Input: part model. Units: mm. Frame: model coordinates. A direction names the side the tool comes from. Round coordinates to 2 decimals unless told otherwise and drop trailing zeros. Loops run counter-clockwise (first coordinate to the right, second up) from the corner with the lowest first, then second, coordinate; pieces in that order, holes last. Notation, with made-up numbers: (84.5, 48.25) -> (125.5, 48.25) arc R13 ccw to (125.5, 57.25) -> close; hole circle Ø1 at (27.25, -1). An arc over 180 degrees is marked (long way). One line per question, with ' | ' between items. Start each with the question number.
Q1. Material intervals for L1, parallel to X at y = 0.55, z = -10.67; L2, parallel to X at y = 1.2, z = -1.5; L3, parallel to Z at x = 25.35, y = 0.6, sorted ascending.
Q2. Mould query, pull axis X, two halves, no side actions, for faces 1 (the face through (-27.5, 0.5, 0.2)), 2 (the face through (-5.5, 1.5, 0.1)), 3 (the face through (0, 2, 0)). Classes: pulls with the +X half, pulls with the -X half, needs draft (parallel to the pull), parting line crosses it, or undercut.
Q3. Access query for faces 4 (the face through (-24.5, 1.5, 3)), 5 (the face through (-0.1, 1.5, -5.5)), 6 (the face through (11.9, 1.5, -4.5)), 7 (the face through (-24.5, 1.5, -3)), 8 (the face through (7.5, 1.5, 0.1)). Directions: +Z, -Z, +X, -X, +Y, -Y. A direction counts if a zero-diameter tool reaches every point of the face in a straight line with its end or side. Return the directions, or none.
Q4. Cut plane A-A on x = 25.35. Return loops of the section in (y, z).
Q5. Contact query for flat-ended pins moving along their axis: P1, Ø0.5, axis at x = 12.5, y = 1.5, coming from the +Z side; P2, Ø0.5, axis at y = 1.5, z = 2.5, coming from the -X side; P3, Ø12, axis at x = -14.5, z = 6.5, coming from the -Y side; P4, Ø0.8, axis at y = 1.5, z = 0.5, coming from the +X side. Output: stop coordinate, or through.
Q6. Cut plane B-B on z = -10.67. Return loops of the section in (x, y).
Q7. Cut plane C-C on x = -4.5. Return loops of the section in (y, z), and give its area (3 significant figures).
Q8. Cut plane D-D on z = 6.5. Return loops of the section in (x, y), and give its area (3 significant figures).
from build123d import *

# Parameters (mm, degrees)
SKETCH_1_W      = 55
SKETCH_1_H      = 25.4
SKETCH_1_R      = 1.1
SKETCH_1_W_2    = 11
SKETCH_1_H_2    = 11
SKETCH_1_W_3    = 9
SKETCH_1_H_3    = 9
SKETCH_1_W_4    = 4
SKETCH_1_H_4    = 6
EXTRUDE_1_DEPTH = 1
SKETCH_1_3_W    = 11
SKETCH_1_3_H    = 11
SKETCH_1_3_W_2  = 9
SKETCH_1_3_H_2  = 9
SKETCH_1_3_W_3  = 4
SKETCH_1_3_H_3  = 6
EXTRUDE_2_DEPTH = 2


with BuildPart() as part:
    # Sketch 1 → Extrude 1 (new body)
    with BuildSketch(Plane(origin=(0, 0, 0), x_dir=(1, 0, 0), z_dir=(0, 1, 0))):
        Rectangle(SKETCH_1_W, SKETCH_1_H)
        with Locations((-19.94, 10.67)):
            Circle(SKETCH_1_R, mode=Mode.SUBTRACT)
        with Locations((25.35, 10.67)):
            Circle(SKETCH_1_R, mode=Mode.SUBTRACT)
        with Locations((25.35, -10.67)):
            Circle(SKETCH_1_R, mode=Mode.SUBTRACT)
        with Locations((-19.94, -10.67)):
            Circle(SKETCH_1_R, mode=Mode.SUBTRACT)
        Rectangle(SKETCH_1_W_2, SKETCH_1_H_2, mode=Mode.SUBTRACT)
        with Locations((12, 0)):
            Rectangle(SKETCH_1_W_3, SKETCH_1_H_3, mode=Mode.SUBTRACT)
        with Locations((-24.5, 0)):
            Rectangle(SKETCH_1_W_4, SKETCH_1_H_4, mode=Mode.SUBTRACT)
    extrude(amount=EXTRUDE_1_DEPTH)

    # Sketch 1_3 → Extrude 2 (add)
    with BuildSketch(Plane(origin=(0, 0, 0), x_dir=(1, 0, 0), z_dir=(0, 1, 0))):
        Rectangle(SKETCH_1_3_W, SKETCH_1_3_H)
        with Locations((12, 0)):
            Rectangle(SKETCH_1_3_W_2, SKETCH_1_3_H_2)
        with Locations((-24.5, 0)):
            Rectangle(SKETCH_1_3_W_3, SKETCH_1_3_H_3)
    extrude(amount=EXTRUDE_2_DEPTH)


solid = part.part
Results:
1) L1: -27.5 to -21.04, -18.84 to 24.25, 26.45 to 27.5 | L2: -26.5 to -22.5, -5.5 to 5.5, 7.5 to 16.5 | L3: -12.7 to -11.77, -9.57 to 9.57, 11.77 to 12.7
2) face 1: pulls with the -X half | face 2: undercut | face 3: needs draft
3) face 4: +Z, -X, +Y | face 5: -Z, +X, -X, +Y | face 6: -Z, +X, +Y | face 7: -Z, -X, +Y | face 8: +Z, -Z, +Y
4) outline: (0, -12.7) -> (1, -12.7) -> (1, -11.77) -> (0, -11.77) -> close; (0, -9.57) -> (1, -9.57) -> (1, 9.57) -> (0, 9.57) -> close; (0, 11.77) -> (1, 11.77) -> (1, 12.7) -> (0, 12.7) -> close
5) P1: z = 4.5 | P2: x = -26.5 | P3: y = 0 | P4: x = 16.5
6) outline: (-27.5, 0) -> (-21.04, 0) -> (-21.04, 1) -> (-27.5, 1) -> close; (-18.84, 0) -> (24.25, 0) -> (24.25, 1) -> (-18.84, 1) -> close; (26.45, 0) -> (27.5, 0) -> (27.5, 1) -> (26.45, 1) -> close
7) outline: (0, -12.7) -> (1, -12.7) -> (1, -5.5) -> (2, -5.5) -> (2, 5.5) -> (1, 5.5) -> (1, 12.7) -> (0, 12.7) -> close | area: 36.4 mm^2
8) outline: (-27.5, 0) -> (27.5, 0) -> (27.5, 1) -> (-27.5, 1) -> close | area: 55.0 mm^2
